Here's how the part is built. I have some questions about the finished solid (model axes, mm). A direction names the side the tool comes from. Round coordinates to 2 decimals unless told otherwise and drop trailing zeros. Loops run counter-clockwise (first coordinate to the right, second up) from the corner with the lowest first, then second, coordinate; pieces in that order, holes last. Notation, with made-up numbers: M 5.5,14 L 62.5,14 A31 cw 62.5,51 Z; hole C -9,3 d3. An arc over 180 degrees is marked long. Answer as a JSON object with one key per item and string values.
from build123d import *

# Parameters (mm, degrees)
F0_W     = 1200
F0_H     = 550
F1_DEPTH = 600
F2_W     = 300
F2_H     = 300
F3_DEPTH = 600.001
F5_DEPTH = 150
F6_R     = 200
F7_DEPTH = 550.001
F9_DEPTH = 600.001


with BuildPart() as f1:
    # F0 (on Front) → F1 (new body)
    with BuildSketch(Plane.XZ):
        Rectangle(F0_W, F0_H)
    extrude(amount=F1_DEPTH)

    # F2 (on face) → F3 (cut, through all)
    with BuildSketch(Plane.XZ.offset(600)):
        with Locations((-450, 125)):
            Rectangle(F2_W, F2_H)
        with Locations((450, 125)):
            Rectangle(F2_W, F2_H)
    extrude(amount=-F3_DEPTH, mode=Mode.SUBTRACT)

    # F4 (on face) → F5 (join)
    with BuildSketch(Plane(origin=(0, 0, 0), x_dir=(-1, 0, 0), z_dir=(0, 1, 0))):
        Polygon((-300, -25), (-300, 275), (-600, -25), align=None)
        Polygon((600, -25), (300, 275), (300, -25), align=None)
    extrude(amount=-F5_DEPTH)

    # F6 (on face) → F7 (cut, through all)
    with BuildSketch(Plane.XY.offset(275)):
        with Locations((0, -300)):
            Circle(F6_R)
    extrude(amount=-F7_DEPTH, mode=Mode.SUBTRACT)

    # F8 (on face) → F9 (cut, through all)
    with BuildSketch(Plane.XZ.offset(600)):
        with BuildLine():
            ThreePointArc((50, -11.6025403784), (86.6025403784, 25), (100, 75))
            ThreePointArc((100, 75), (-50, 161.6025403784), (-50, -11.6025403784))
            Line((-50, -11.6025403784), (-50, 75))
            Line((-50, 75), (50, 75))
            Line((50, 75), (50, -11.6025403784))
        make_face()
        with BuildLine():
            Line((-50, 75), (-50, -11.6025403784))
            ThreePointArc((-50, -11.6025403784), (0, -25), (50, -11.6025403784))
            Line((50, -11.6025403784), (50, 75))
            Line((50, 75), (-50, 75))
        make_face()
        with BuildLine():
            ThreePointArc((50, -11.6025403784), (0, -25), (-50, -11.6025403784))
            Line((-50, -11.6025403784), (-50, -625))
            Line((-50, -625), (50, -625))
            Line((50, -625), (50, -11.6025403784))
        make_face()
    extrude(amount=-F9_DEPTH, mode=Mode.SUBTRACT)


solid = f1.part
Item 1: We'd pull the mould along X, two halves only. Please class faces 1 (the face through (-452, -74, 123)), 2 (the face through (448, -74, 127)), 3 (the face through (382, -296, -275)), 4 (the face through (-50, -54, -141)): +X half, -X half, draft (parallel to the pull), parting line (faces both ways), or undercut.
Solution:
{"face 1": "-X half", "face 2": "+X half", "face 3": "draft", "face 4": "undercut"}
Item 2: If I drill on L1, parallel to X at y = -536, z = -31.5; L2, parallel to X at y = -553, z = 75; L3, parallel to Z at x = 369, y = -243.5, over which ranges is the centre line in solid material (lowest first)? Write a range as from..to.
Solution:
{"L1": "x = -600..-50, 50..600", "L2": "x = -300..-100, 100..300", "L3": "z = -275..-25"}
Item 3: I want a section at A-A on z = -182.5. List the corners of the cut face in (x, y) for me, plus the area to 3 significant figures.
Solution:
{"outline": "M -600,-600 L -50,-600 L -50,-493.65 A200 cw -50,-106.35 L -50,0 L -600,0 Z; M 50,-600 L 600,-600 L 600,0 L 50,0 L 50,-106.35 A200 cw 50,-493.65 Z", "area": "574,000 mm2"}
Item 4: I want a section at D-D on x = -457. List the corners of the cut face in (y, z) for me.
Solution:
{"outline": "M -600,-275 L 0,-275 L 0,118 L -150,118 L -150,-25 L -600,-25 Z"}
Item 5: I want a section at B-B on x = 0. List the corners of the cut face in (y, z) for me, plus the area to 3 significant figures.
Solution:
{"outline": "M -600,175 L -500,175 L -500,275 L -600,275 Z; M -100,175 L 0,175 L 0,275 L -100,275 Z", "area": "20,000 mm2"}
Item 6: I want a section at C-C on y = -300. List the corners of the cut face in (x, z) for me, plus the area to 3 significant figures.
Solution:
{"outline": "M -600,-275 L -200,-275 L -200,275 L -300,275 L -300,-25 L -600,-25 Z; M 200,-275 L 600,-275 L 600,-25 L 300,-25 L 300,275 L 200,275 Z", "area": "260,000 mm2"}
Item 7: For P1, Ø3, axis at y = -409.5, z = 68, coming from the -X side, with a flat end and sliding along its axis, tell me the tip position at first contact or that it passes through.
Solution:
{"P1": "stops at x = -300"}
Item 8: For faces 5 (the face through (300, -378, 123)), 6 (the face through (-600, -296, -152)), 7 (the face through (-300, -378, 123)), 8 (the face through (600, -296, -152)), 9 (the face through (-50, -548, -141)), which set-ups out of +Z, -Z, +X, -X, +Y, -Y let a thin tool reach every point of the face, with its end or its side?
Solution:
{"face 5": "+Z, +X, -Y", "face 6": "+Z, -Z, -X, +Y, -Y", "face 7": "+Z, -X, -Y", "face 8": "+Z, -Z, +X, +Y, -Y", "face 9": "-Z, +Y, -Y"}
